Verification items for this drawing (mm, ordinates from the low corner). A direction names the side the tool comes from. Give positions to 0.01 mm unless a question says otherwise; leave off trailing zeros. Loops run counter-clockwise (first coordinate to the right, second up) from the corner with the lowest first, then second, coordinate; pieces in that order, holes last. Notation, with made-up numbers: (-38.5, 22.5) -> (-24.5, 22.5) arc R16 ccw to (-24.5, 48.5) -> close; hole circle Ø8 at (13.5, 45.25). An arc over 180 degrees is marked (long way). Write each question's results on one line, items separated by ' | '. Start each with the question number.
1) Scan lines: line 1 (Y direction, x = 12, z = 167); line 2 (Y direction, x = 160.5, z = 34); line 3 (X direction, y = 127, z = 72.5). Record each from-to range of solid material in increasing order. Write a range as from..to.
2) Sectioned sample at B-B on z = 78. Record the cut outline in (x, y).
3) Sectioned sample at C-C on y = 73. Record the cut outline in (x, z).
4) Sectioned sample at D-D on z = 182. Record the cut outline in (x, y), then the cut area to 3 significant figures.
5) Draft check along Y on the marked faces 4, 5, 6 and 7. Enter one of: pulls with the +Y half, pulls with the -Y half, needs draft (parallel to the pull), parting line crosses it, or undercut.
6) Set-up check for the marked faces 1, 2 and 3: record each of +Z, -Z, +X, -X, +Y, -Y from which the full face is reachable in a straight line by a thin tool's end or side.
7) Depth check by flat-ended pin: pin 1 (5 mm diameter, centred on y = 107.5, z = 100.5, fed in from -X); pin 2 (4 mm diameter, centred on x = 72.5, z = 114, fed in from +Y); pin 3 (4 mm diameter, centred on x = 72, y = 110, fed in from -Z). Enter the tip coordinate at first touch or a pass-through.
8) Sectioned sample at A-A on x = 190.5. Record the cut outline in (y, z), then the cut area to 4 significant figures.
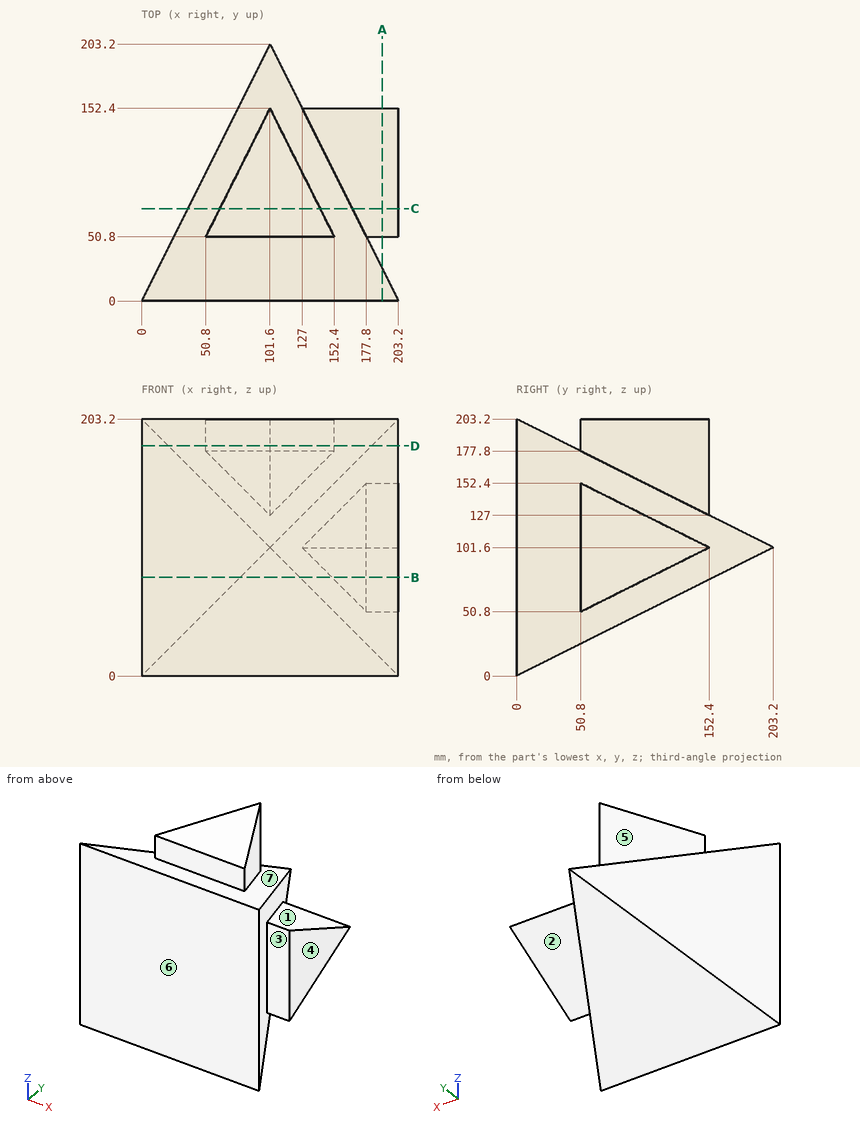
Result:
1) line 1: 0..24 | line 2: 0..68 | line 3: 63.5..139.7
2) outline: (0, 0) -> (203.2, 0) -> (177.8, 50.8) -> (203.2, 50.8) -> (203.2, 105.2) -> (150.6, 105.2) -> (125.2, 156) -> (78, 156) -> close
3) outline: (36.5, 36.5) -> (166.7, 36.5) -> (166.7, 61.9) -> (203.2, 61.9) -> (203.2, 141.3) -> (166.7, 141.3) -> (166.7, 166.7) -> (141.3, 166.7) -> (141.3, 203.2) -> (61.9, 203.2) -> (61.9, 166.7) -> (36.5, 166.7) -> close
4) outline: (0, 0) -> (203.2, 0) -> (182, 42.4) -> (21.2, 42.4) -> close; (50.8, 50.8) -> (152.4, 50.8) -> (101.6, 152.4) -> close | area: 12,900 mm^2
5) face 4: needs draft | face 5: pulls with the +Y half | face 6: pulls with the -Y half | face 7: undercut
6) face 1: +Z, +X, +Y | face 2: -Z, +X, +Y | face 3: +Z, -Z, +X
7) pin 1: x = 52.5 | pin 2: y = 149 | pin 3: z = 54
8) outline: (0, 0) -> (25.4, 12.7) -> (25.4, 190.5) -> (0, 203.2) -> close; (50.8, 50.8) -> (152.4, 101.6) -> (50.8, 152.4) -> close | area: 10,000 mm^2
